Work out the finished part from the listing and answer in its coordinate system (mm). Coordinates: 2 decimals unless noted, no trailing zeros. Loops run counter-clockwise (first coordinate to the right, second up) from the corner with the lowest first, then second, coordinate; pieces in that order, holes last. Notation, with made-up numbers: (18.5, -19) - (53.5, -19) arc R22 cw to (53.5, -2) - close; hole circle Ø11 at (49.25, -8). An arc over 180 degrees is marked (long way). Write each question's results on one line, items separated by ' | '. Start each with the question number.
Item 1: Section C-C, the plane z = -3.5 is taken. Write down the section's boundary in (x, y).
Item 2: Section A-A, the plane z = 0 is taken. Write down the section's boundary in (x, y), plus the area to 3 significant figures.
Item 3: Each of these flat-tipped pins is pushed along its axis until it touches: pin 1 Ø5 at (x, z) = (2, -4.5) entering from -Y; pin 2 Ø1.5 at (y, z) = (2, -5.5) entering from +X; pin 3 Ø1.5 at (y, z) = (2.5, -6.5) entering from +X. Where does it stop, or does it pass through?
Item 4: For a pull along Z with two mould halves and no side action, classify faces 1 (the face through (-14.985, 0.042, -0.66)), 2 (the face through (4, 3, 4)), 3 (the face through (-4.88, -0.04, 1.08)) as +Z half, -Z half, draft (parallel to the pull), parting line (faces both ways), or undercut.
Item 5: Consider probe 1 along Z at (x, y) = (0, 1.1); probe 2 along Z at (x, y) = (3, -1); probe 3 along X at (y, z) = (-2.15, -12.5). Determine where each line is inside the solid, lowest interval first. Write a range as [from, to].
Item 6: Section D-D, the plane y = -2.1 is taken. Write down the section's boundary in (x, z), plus the area to 3 significant figures.
Item 7: Section B-B, the plane x = 10 is taken. Write down the section's boundary in (y, z), plus the area to 3 significant figures.
Solid Edge part; units mm, degrees
sketch "Sketch1" plane through (0, 0, 0) normal (0, -1, 0) x (1, 0, 0)
  circle A0 centre (0, 0) radius 15
extrude "Protrusion1" add sketch "Sketch1" along normal mid plane 6
hole "Bohrung_1" at (0, -3, 0) direction (0, 1, 0) diameter 10 end through all
hole "Bohrung_2" at (10, -3, 0) direction (0, 1, 0) diameter 1 end up to next
pattern_circular "Pattern1" count 3 over 360 about axis through (0, -3, 0) along (0, -1, 0) of "Bohrung_2"
properties part number "DV2" material "Grauguss 20"
Answer key:
1) outline: (-14.59, -3) - (-3.57, -3) - (-3.57, 3) - (-14.59, 3) - close; (3.57, -3) - (14.59, -3) - (14.59, 3) - (3.57, 3) - close
2) outline: (-15, -3) - (-5, -3) - (-5, 3) - (-15, 3) - close; (5, -3) - (9.5, -3) - (9.5, 3) - (5, 3) - close; (10.5, -3) - (15, -3) - (15, 3) - (10.5, 3) - close | area: 114 mm^2
3) pin 1: stops at y = -3 | pin 2: stops at x = 14.23 | pin 3: stops at x = 13.85
4) face 1: parting line | face 2: draft | face 3: undercut
5) probe 1: z = [-15, -5], [5, 15] | probe 2: z = [-14.7, -4], [4, 14.7] | probe 3: x = [-8.29, 8.29]
6) outline: circle Ø30 at (0, 0); hole circle Ø1 at (-5, -8.66); hole circle Ø1 at (-5, 8.66); hole circle Ø10 at (0, 0); hole circle Ø1 at (10, 0) | area: 626 mm^2
7) outline: (-3, -11.18) - (3, -11.18) - (3, -0.5) - (-3, -0.5) - close; (-3, 0.5) - (3, 0.5) - (3, 11.18) - (-3, 11.18) - close | area: 128 mm^2
